For this review, take the finished solid that the model builds, in its own axes (mm). Face numbers are marked on the shaded views. A direction names the side the tool comes from. Coordinates: 2 decimals unless noted, no trailing zeros. Loops run counter-clockwise (first coordinate to the right, second up) from the corner with the lowest first, then second, coordinate; pieces in that order, holes last. Notation, with made-up numbers: M 24.5,-14 L 35.5,-14 A23 cw 35.5,7 Z; hole C 85.25,12 d7. An arc over 180 degrees is marked long. Write item = value, one per line.
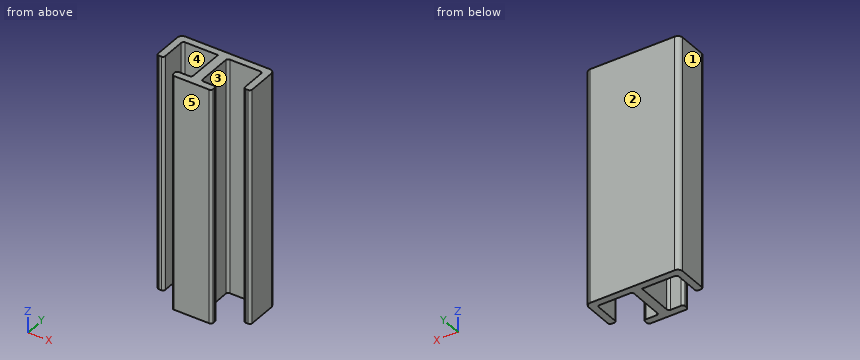
from build123d import *

# Parameters (mm, degrees)
F1_DEPTH = 100
F2_R     = 2
F3_R     = 1


with BuildPart() as f1:
    # F0 (on Top) → F1 (new body)
    with BuildSketch(Plane.XY):
        Polygon((20, 10), (-20, 10), (-20, -5), (-17, -5), (-17, 7), (-2, 7), (-2, -9.5), (-8.5, -9.5), (-8.5, -12.5), (0, -12.5), (8.5, -12.5), (8.5, -9.5), (2, -9.5), (2, 7), (17, 7), (17, -5), (20, -5), align=None)
    extrude(amount=F1_DEPTH)

    # F2
    f2_edges = [f1.edges().sort_by_distance(p)[0] for p in [
        (-20, 10, 50),
        (20, 10, 50),
    ]]
    fillet(f2_edges, radius=F2_R)

    # F3
    f3_edges = [f1.edges().sort_by_distance(p)[0] for p in [
        (-17, -5, 50),
        (-20, -5, 50),
        (-17, 7, 50),
        (2, 7, 50),
        (8.5, -12.5, 50),
        (8.5, -9.5, 50),
        (-8.5, -12.5, 50),
        (-8.5, -9.5, 50),
        (-2, -9.5, 50),
        (2, -9.5, 50),
        (17, -5, 50),
        (20, -5, 50),
        (17, 7, 50),
    ]]
    fillet(f3_edges, radius=F3_R)


solid = f1.part
Q1. Add section A-A (x = -6.5). Write out the cut boundary in (y, z), and give its area (3 significant figures).
Solved:
outline = M -12.5,0 L -9.5,0 L -9.5,100 L -12.5,100 Z; M 7,0 L 10,0 L 10,100 L 7,100 Z
area = 600 mm²
Q2. Machinability: for the marked faces 4 and 5, which of the approach directions +Z, -Z, +X, -X, +Y, -Y give a long, thin tool a straight path to every point of the face, cutting with its end or side? Answer none if there is none.
Solved:
face_4 = +Z, -Z
face_5 = +Z, -Z, +X, -X, -Y
Q3. For pin 1 Ø0.8 at (y, z) = (-11, 56.5) entering from +X; pin 2 Ø0.8 at (x, z) = (-18.5, 56) entering from -Y; pin 3 Ø0.5 at (y, z) = (-11, 44) entering from -X; pin 4 Ø3 at (x, y) = (5, -5.5) entering from -Z, all flat-tipped, find the tip position at first contact; note any pin that passes through.
Solved:
pin_1 = 8.5
pin_2 = -5
pin_3 = -8.5
pin_4 = through
Q4. Add section D-D (x = 14.5). Write out the cut boundary in (y, z), and give its area (3 significant figures).
Solved:
outline = M 7,0 L 10,0 L 10,100 L 7,100 Z
area = 300 mm²
Q5. For line 1 along X through (y, z) = (0.75, 39.5); line 2 along Y through (x, z) = (6, 44.5); line 3 along X through (y, z) = (-6, 85.5), list the stretches that pass through material, from the lowest coordinate up.
Solved:
line_1 = -20 to -17, -2 to 2, 17 to 20
line_2 = -12.5 to -9.5, 7 to 10
line_3 = -2 to 2
Q6. Draft analysis for pull direction X (two halves, no side actions). For the marked faces 1, 2 and 3, state which applies: +X half, -X half, draft (parallel to the pull), parting line (faces both ways), or undercut.
Solved:
face_1 = -X half
face_2 = draft
face_3 = undercut
Q7. Add section C-C (y = -6.75). Write out the cut boundary in (x, z), and give its area (3 significant figures).
Solved:
outline = M -2,0 L 2,0 L 2,100 L -2,100 Z
area = 400 mm²
